from build123d import *

# Parameters (mm, degrees)
ESQUISSE1_R        = 10
ESQUISSE1_R_2      = 0.75
BOSS_EXTRU_1_DEPTH = 2.75
CHANFREIN1_SIZE    = 0.49
CHANFREIN2_SIZE    = 0.49
ESQUISSE2_R        = 1.5
BOSS_EXTRU_2_DEPTH = 8.5


with BuildPart() as part:
    # Esquisse1 → Boss.-Extru.1 (new, symmetric)
    with BuildSketch(Plane.XY):
        with BuildLine():
            Line((5.5, -3.5), (5.5, 0.5))
            ThreePointArc((5.5, 0.5), (8.157393572, 4.917261043), (13.304878049, 4.639161646))
            ThreePointArc((13.304878049, 4.639161646), (37.430230582, 18.939570643), (11.039844892, 28.430717857))
            Line((11.039844892, 28.430717857), (-2.571067812, 14.819805153))
            ThreePointArc((-2.571067812, 14.819805153), (-4.738795325, 11.575571665), (-5.5, 7.748737342))
            Line((-5.5, 7.748737342), (-5.5, -3.5))
            ThreePointArc((-5.5, -3.5), (0, -9), (5.5, -3.5))
        make_face()
        with Locations((22, 17.470562748)):
            Circle(ESQUISSE1_R, mode=Mode.SUBTRACT)
        with Locations((0, -7.25)):
            Circle(ESQUISSE1_R_2, mode=Mode.SUBTRACT)
        with BuildLine():
            Line((2, 3.5), (2, -3.5))
            ThreePointArc((2, -3.5), (0, -5.5), (-2, -3.5))
            Line((-2, -3.5), (-2, 3.5))
            ThreePointArc((-2, 3.5), (0, 5.5), (2, 3.5))
        make_face(mode=Mode.SUBTRACT)
    extrude(amount=BOSS_EXTRU_1_DEPTH, both=True)

    # Chanfrein1
    chanfrein1_edges = [part.edges().sort_by_distance(p)[0] for p in [
        (0, 5.5, 2.75),
        (-2, 0, 2.75),
        (0, -5.5, 2.75),
        (2, 0, 2.75),
        (-0.75, -7.25, 2.75),
    ]]
    chamfer(chanfrein1_edges, length=CHANFREIN1_SIZE)

    # Chanfrein2
    chanfrein2_edges = [part.edges().sort_by_distance(p)[0] for p in [
        (0, 5.5, -2.75),
        (-2, 0, -2.75),
        (0, -5.5, -2.75),
        (2, 0, -2.75),
        (-0.75, -7.25, -2.75),
    ]]
    chamfer(chanfrein2_edges, length=CHANFREIN2_SIZE)

    # Esquisse2 → Boss.-Extru.2 (add, symmetric)
    with BuildSketch(Plane.XY):
        with Locations(Location((0, 7.49, 0), (0, 0, 270.000522617))):
            Circle(ESQUISSE2_R)
    extrude(amount=BOSS_EXTRU_2_DEPTH, both=True)


solid = part.part
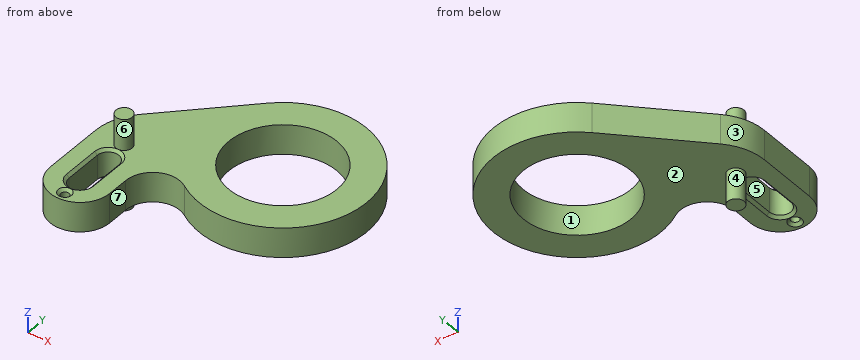
Could you check a few things on this model? Use its own coordinates, in mm. Face numbers are marked on the shaded views. A direction names the side the tool comes from. Round coordinates to 2 decimals unless told otherwise and drop trailing zeros. Order: outer loops, then holes, each group sorted by start corner. A loop starts at its lowest first (then second) coordinate and runs counter-clockwise, first axis right, second up. Notation, with made-up numbers: M -34,-21 L -22,-21 A25 ccw -22,17 Z; hole C -31,77.5 d8. An arc over 180 degrees is marked long. One line per item, written item: value.
(1) If we mould it in two halves opening along X, with no side actions, what happens to the marked faces 1, 2 and 3? For each: released by +X, released by -X, zero draft, split by the parting line, or undercut.
Ans:
face 1: undercut
face 2: zero draft
face 3: released by -X
(2) I'm going to push flat-ended pins straight in: P1, Ø1.2, axis at y = -2, z = -1, coming from the +X side; P2, Ø6, axis at x = 12.5, z = 2, coming from the +Y side; P3, Ø10, axis at x = 33, y = 13.5, coming from the -Z side. Where does each tip first touch, or does it pass through?
Ans:
P1: stops at x = 5.5
P2: stops at y = 31.54
P3: stops at z = -2.75
(3) Imagine slicing it at C-C (y = 10.5). Write out the boundary of the cut face in (x, z), and give its area (3 significant figures).
Ans:
outline: M -5.11,-2.75 L 14.83,-2.75 L 14.83,2.75 L -5.11,2.75 Z; M 29.17,-2.75 L 35.84,-2.75 L 35.84,2.75 L 29.17,2.75 Z
area: 146 mm^2
(4) I need wall thicknesses on line 1 along Y through (x, z) = (22, -0.6); line 2 along Z through (x, y) = (9.5, 8.5); line 3 along Y through (x, z) = (25, -2). Which ranges of each line are inside material? Lowest first, please. Write a range as from..to.
Ans:
line 1: y = 1.97..7.47, 27.47..32.97
line 2: z = -2.75..2.75
line 3: y = 2.26..7.93, 27.01..32.68
(5) Imagine slicing it at D-D (z = 7.75). Write out the boundary of the cut face in (x, y), and give its area (3 significant figures).
Ans:
outline: C 0,7.49 d3
area: 7.07 mm^2
(6) Imagine slicing it at A-A (y = -2.5). Write out the boundary of the cut face in (x, z), and give its area (3 significant figures).
Ans:
outline: M -5.5,-2.75 L -2.49,-2.75 L -2,-2.26 L -2,2.26 L -2.49,2.75 L -5.5,2.75 Z; M 2,-2.26 L 2.49,-2.75 L 5.5,-2.75 L 5.5,2.75 L 2.49,2.75 L 2,2.26 Z
area: 38.0 mm^2
(7) Imagine slicing it at B-B (x = 22). Write out the boundary of the cut face in (y, z), and give its area (3 significant figures).
Ans:
outline: M 1.97,-2.75 L 7.47,-2.75 L 7.47,2.75 L 1.97,2.75 Z; M 27.47,-2.75 L 32.97,-2.75 L 32.97,2.75 L 27.47,2.75 Z
area: 60.5 mm^2
(8) Which directions (+Z, -Z, +X, -X, +Y, -Y) give clear straight access to the entire face, cutting with the end or side of a thin tool? Please do the marked faces 4, 5, 6 and 7.
Ans:
face 4: -Z
face 5: +Z, -Z
face 6: +Z
face 7: +Z, -Z, +X, -Y
